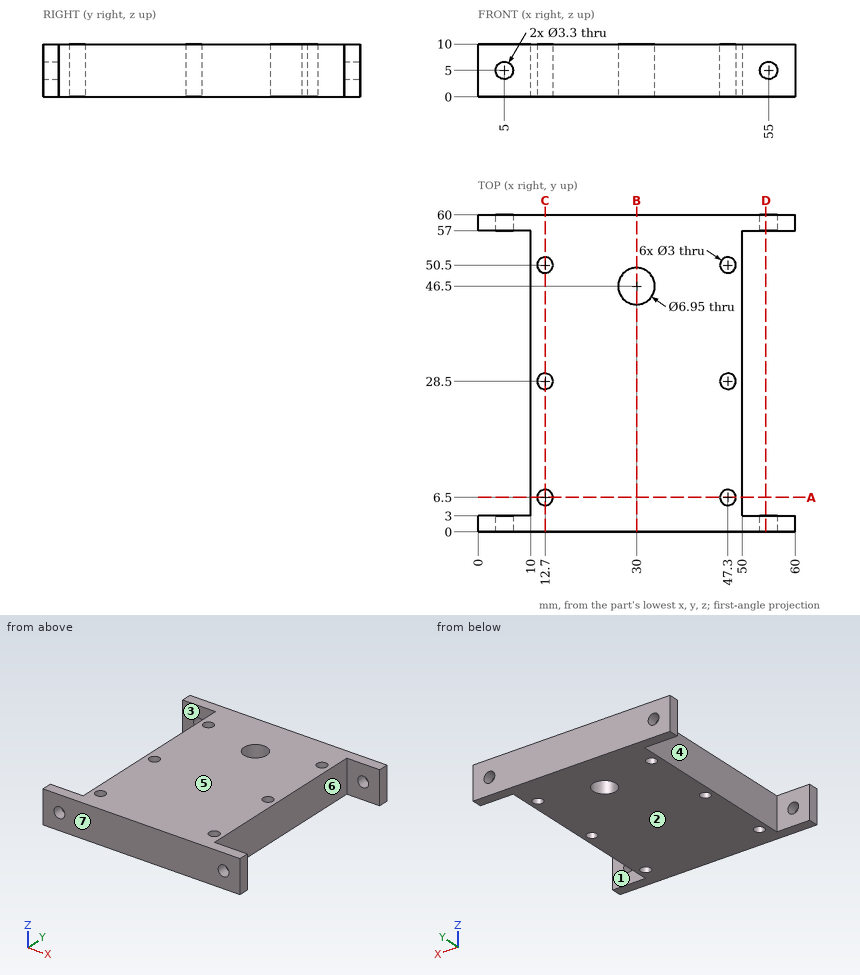
Job drawing, mm, ordinate dimensions from the low corner. One solid piece. A direction names the side the tool comes from. Give positions to 0.01 mm unless a question says otherwise; leave off trailing zeros. Loops run counter-clockwise (first coordinate to the right, second up) from the corner with the lowest first, then second, coordinate; pieces in that order, holes last. Notation, with made-up numbers: M -27.75,26.5 L 30.25,26.5 A14 ccw 30.25,32.5 Z; hole C 73.25,5.5 d3. An arc over 180 degrees is marked long. Answer in a Markdown table with one row per item. Add a question column.
Item 1: Drop a flat-ended pin along its axis: P1, Ø5, axis at y = 41.5, z = 6, coming from the +X side. Give the stop position or say it passes through.
Item 2: Tool access for the marked faces 1, 2 and 3: list every direction of +Z, -Z, +X, -X, +Y, -Y with a clear straight run to the whole face (end or side of a thin tool).
Item 3: Band-saw the part on A-A on y = 6.5. Give the cut face in (x, z), then the cut area to 3 significant figures.
Item 4: Probe probe 1 along Y at (x, z) = (47.3, 2.75); probe 2 along X at (y, z) = (59.1, 5); probe 3 along Y at (x, z) = (51.5, 1.25). List the from-to ranges inside material, lowest first.
Item 5: Mould opens along Y. For the marked faces 4, 5, 6 and 7 say: +Y half, -Y half, draft (parallel to the pull), parting line (faces both ways), or undercut.
Item 6: Band-saw the part on D-D on x = 54.5. Give the cut face in (y, z).
Item 7: Band-saw the part on C-C on x = 12.7. Give the cut face in (y, z), then the cut area to 3 significant figures.
Item 8: Band-saw the part on B-B on x = 30. Give the cut face in (y, z) (3 decimals), then the cut area to 4 significant figures.
Reply:
| question | item | result |
|---|---|---|
| 1 | P1 | stops at x = 50 |
| 2 | face 1 | +Z, -Z, +X |
| 2 | face 2 | -Z, +X, -X, +Y, -Y |
| 2 | face 3 | +Z, -Z, -X |
| 3 | outline | M 10,0 L 11.2,0 L 11.2,10 L 10,10 Z; M 14.2,0 L 45.8,0 L 45.8,10 L 14.2,10 Z; M 48.8,0 L 50,0 L 50,10 L 48.8,10 Z |
| 3 | area | 340 mm^2 |
| 4 | probe 1 | y = 0 to 5, 8 to 27, 30 to 49, 52 to 60 |
| 4 | probe 2 | x = 0 to 3.35, 6.65 to 53.35, 56.65 to 60 |
| 4 | probe 3 | y = 0 to 3, 57 to 60 |
| 5 | face 4 | undercut |
| 5 | face 5 | draft |
| 5 | face 6 | undercut |
| 5 | face 7 | -Y half |
| 6 | outline | M 0,0 L 3,0 L 3,3.43 L 0,3.43 Z; M 0,6.57 L 3,6.57 L 3,10 L 0,10 Z; M 57,0 L 60,0 L 60,3.43 L 57,3.43 Z; M 57,6.57 L 60,6.57 L 60,10 L 57,10 Z |
| 7 | outline | M 0,0 L 5,0 L 5,10 L 0,10 Z; M 8,0 L 27,0 L 27,10 L 8,10 Z; M 30,0 L 49,0 L 49,10 L 30,10 Z; M 52,0 L 60,0 L 60,10 L 52,10 Z |
| 7 | area | 510 mm^2 |
| 8 | outline | M 0,0 L 43.025,0 L 43.025,10 L 0,10 Z; M 49.975,0 L 60,0 L 60,10 L 49.975,10 Z |
| 8 | area | 530.5 mm^2 |
